```python
from build123d import *

# Parameters (mm, degrees)
SKETCH1_W           = 100
SKETCH1_H           = 331
BOSS_EXTRUDE1_DEPTH = 10
SKETCH2_R           = 10
SKETCH2_R_2         = 2.5
SKETCH2_R_3         = 17
SKETCH2_R_4         = 1.5
CUT_EXTRUDE1_DEPTH  = 311.286961886
SKETCH3_R           = 2
CUT_EXTRUDE2_DEPTH  = 15


with BuildPart() as part:
    # Sketch1 → Boss-Extrude1 (new body)
    with BuildSketch(Plane(origin=(0, 0, 0), x_dir=(1, 0, 0), z_dir=(0, 1, 0))):
        with Locations((-29.223933498, -134.335900248)):
            Rectangle(SKETCH1_W, SKETCH1_H)
    extrude(amount=BOSS_EXTRUDE1_DEPTH)

    # Sketch2 → Cut-Extrude1 (cut, through all)
    with BuildSketch(Plane(origin=(0, 10, 0), x_dir=(1, 0, 0), z_dir=(0, 1, 0))):
        with Locations(Location((-49.223933498, -2.835900248, 0), (0, 0, 270))):
            Circle(SKETCH2_R)
        with Locations(Location((-73.223933498, -2.835900248, 0), (0, 0, 270))):
            Circle(SKETCH2_R_2)
        with Locations(Location((-25.223933498, -2.835900248, 0), (0, 0, 270))):
            Circle(SKETCH2_R_2)
        with Locations(Location((-49.223933498, -104.835900248, 0), (0, 0, 270))):
            Circle(SKETCH2_R)
        with Locations(Location((-73.223933498, -104.835900248, 0), (0, 0, 270))):
            Circle(SKETCH2_R_2)
        with Locations(Location((-25.223933498, -104.835900248, 0), (0, 0, 270))):
            Circle(SKETCH2_R_2)
        with Locations(Location((-49.223933498, -53.835900248, 0), (0, 0, 270))):
            Circle(SKETCH2_R_3)
        with Locations(Location((-64.073175903, -38.986657843, 0), (0, 0, 270))):
            Circle(SKETCH2_R_4)
        with Locations(Location((-34.374691094, -38.986657843, 0), (0, 0, 270))):
            Circle(SKETCH2_R_4)
        with Locations(Location((-34.374691094, -68.685142653, 0), (0, 0, 270))):
            Circle(SKETCH2_R_4)
        with Locations(Location((-64.073175903, -68.685142653, 0), (0, 0, 270))):
            Circle(SKETCH2_R_4)
    extrude(amount=-CUT_EXTRUDE1_DEPTH, mode=Mode.SUBTRACT)

    # Sketch3 → Cut-Extrude2 (cut)
    with BuildSketch(Plane.XY.offset(299.835900248)):
        with Locations((-59.223933498, 5)):
            Circle(SKETCH3_R)
        with Locations((0.776066502, 5)):
            Circle(SKETCH3_R)
    extrude(amount=-CUT_EXTRUDE2_DEPTH, mode=Mode.SUBTRACT)


solid = part.part
```
Geometry check sheet. Reference: the model listing, model coordinates, mm. Round coordinates to 2 decimals unless told otherwise and drop trailing zeros. Loops run counter-clockwise (first coordinate to the right, second up) from the corner with the lowest first, then second, coordinate; pieces in that order, holes last. Notation, with made-up numbers: (67, -24.5) - (85, -24.5) arc R24 ccw to (85, -1.5) - close; hole circle Ø7 at (-36.5, 82.5). An arc over 180 degrees is marked (long way). Use a Markdown table: item, result.
Q1. Go/stop test with flat-tipped pins: P1, Ø3.5, axis at x = -34.37, z = 68.69, coming from the -Y side; P2, Ø3, axis at x = -59.22, y = 5, coming from the +Z side. Record where each tip stops, or that it passes through.
Solutions:
| item | result |
|---|---|
| P1 | stops at y = 0 |
| P2 | stops at z = 284.84 |
Q2. Draft check along Z on faces 1 (the flat face through (20.776, 5, 137)), 2 (the flat face through (-30, 5, -31.164)), 3 (the cylindrical face through (-37.73, 5.07, 41.31)). Enter one of: released by +Z, released by -Z, zero draft, split by the parting line, or undercut.
Solutions:
| item | result |
|---|---|
| face 1 | zero draft |
| face 2 | released by -Z |
| face 3 | undercut |
Q3. Cross-section at B-B on z = 111. Record the cut outline in (x, y), plus the area to 3 significant figures.
Solutions:
| item | result |
|---|---|
| outline | (-79.22, 0) - (-57.1, 0) - (-57.1, 10) - (-79.22, 10) - close; (-41.35, 0) - (20.78, 0) - (20.78, 10) - (-41.35, 10) - close |
| area | 843 mm2 |
Q4. Material ranges on line 1 (Z direction, x = -25.5, y = 6.25); line 2 (Z direction, x = -71, y = 2); line 3 (Z direction, x = -56.5, y = 2.75), recorded low to high.
Solutions:
| item | result |
|---|---|
| line 1 | z = -31.16 to 0.35, 5.32 to 102.35, 107.32 to 299.84 |
| line 2 | z = -31.16 to 1.69, 3.98 to 103.69, 105.98 to 299.84 |
| line 3 | z = -31.16 to -4.02, 9.7 to 38.47, 69.2 to 97.98, 111.7 to 299.84 |
Q5. Cross-section at C-C on y = 5. State how many separate pieces and enclosed holes the cut face has, plus the area to 3 significant figures.
Solutions:
| item | result |
|---|---|
| separate pieces | 1 |
| enclosed holes | 11 |
| area | 31,300 mm2 |
Q6. Cross-section at A-A on x = -52. Record the cut outline in (y, z), plus the area to 3 significant figures.
Solutions:
| item | result |
|---|---|
| outline | (0, -31.16) - (10, -31.16) - (10, -6.77) - (0, -6.77) - close; (0, 12.44) - (10, 12.44) - (10, 37.06) - (0, 37.06) - close; (0, 70.61) - (10, 70.61) - (10, 95.23) - (0, 95.23) - close; (0, 114.44) - (10, 114.44) - (10, 299.84) - (0, 299.84) - close |
| area | 2,590 mm2 |
